```python
from build123d import *

# Parameters (mm, degrees)
SKETCH1_W                  = 44.45
SKETCH1_H                  = 44.45
BOSS_EXTRUDE1_DEPTH        = 9.525
CBORE_FOR_1_4_1_AT_2_COUNT = 2
CBORE_FOR_1_4_1_AT_2_PITCH = 45.963472584
CBORE_FOR_1_4_1_AT_3_COUNT = 2
CBORE_FOR_1_4_1_AT_3_PITCH = 32.501083151
SKETCH6_R                  = 6.35
CUT_EXTRUDE1_DEPTH         = 4.7752
SKETCH7_R                  = 2.38125
CUT_EXTRUDE2_DEPTH         = 33.842455374


with BuildPart() as part:
    # Sketch1 → Boss-Extrude1 (new body)
    with BuildSketch(Plane.XY):
        Rectangle(SKETCH1_W, SKETCH1_H)
    extrude(amount=BOSS_EXTRUDE1_DEPTH)

    # Sketch5 → CBORE for 1/4 _1 (revolve, cut)
    with BuildSketch(Plane(origin=(-15.875, 16.626083151, 0), x_dir=(0, 1, 0), z_dir=(1, 0, 0))):
        Polygon((0, 0), (0, 9.525), (3.175, 9.525), (3.175, 0.508), (3.81, 0.508), (3.81, 0.127), (3.937, 0), align=None)
    cbore_for_1_4_1 = revolve(axis=Axis((-15.875, 16.626083151, -6.35), (0, 0, 1)), mode=Mode.SUBTRACT)

    # CBORE for 1/4 _1 at 2: CBORE for 1/4 _1 ×2
    with Locations(*[Vector(0.7071067811865476, -0.7071067811865476, 0) * (i * CBORE_FOR_1_4_1_AT_2_PITCH) for i in range(1, CBORE_FOR_1_4_1_AT_2_COUNT)]):
        add(cbore_for_1_4_1, mode=Mode.SUBTRACT)

    # CBORE for 1/4 _1 at 3: CBORE for 1/4 _1 ×2
    with Locations(*[(0, -i * CBORE_FOR_1_4_1_AT_3_PITCH, 0) for i in range(1, CBORE_FOR_1_4_1_AT_3_COUNT)]):
        add(cbore_for_1_4_1, mode=Mode.SUBTRACT)

    # Sketch6 → Cut-Extrude1 (cut)
    with BuildSketch(Plane(origin=(0, 0, 0), x_dir=(-1, 0, 0), z_dir=(0, 0, -1))):
        with Locations((6.355653141, -6.355653141)):
            Circle(SKETCH6_R)
    extrude(amount=-CUT_EXTRUDE1_DEPTH, mode=Mode.SUBTRACT)

    # Sketch7 → Cut-Extrude2 (cut, through all)
    with BuildSketch(Plane(origin=(0, 0, 0), x_dir=(-1, 0, 0), z_dir=(0, 0, -1))):
        with Locations((6.355653141, -6.355653141)):
            Circle(SKETCH7_R)
    extrude(amount=-CUT_EXTRUDE2_DEPTH, mode=Mode.SUBTRACT)


solid = part.part
```
Here's how the part is built. I have some questions about the finished solid (model axes, mm). A direction names the side the tool comes from. Give positions to 0.01 mm unless a question says otherwise; leave off trailing zeros. Loops run counter-clockwise (first coordinate to the right, second up) from the corner with the lowest first, then second, coordinate; pieces in that order, holes last. Notation, with made-up numbers: M -22,32 L 35,32 A5 cw 35,40 Z; hole C -33,48.25 d10. An arc over 180 degrees is marked long. Return JSON: item names as keys, results as strings.
Item 1: On a 3-axis mill with a long thin cutter (end or side, diameter ignored), from which of +Z, -Z, +X, -X, +Y, -Y can I reach the whole of each face in a straight line? I mean faces 1 (the flat face through (14, -18, 0.508)), 2 (the flat face through (0, 0, 9.525)). Say none if no direction works.
A:
{"face 1": "-Z", "face 2": "+Z, +X, -X, +Y, -Y"}
Item 2: Please list where these lines run through material, in increasing order: line 1 (Y direction, x = -14, z = 2.75) (3 decimals); line 2 (Y direction, x = -17, z = 2) (3 decimals); line 3 (Y direction, x = 16.5, z = 1) (1 decimal).
A:
{"line 1": "y = -22.225 to -18.437, -13.313 to 14.064, 19.188 to 22.225", "line 2": "y = -22.225 to -18.844, -12.906 to 13.657, 19.595 to 22.225", "line 3": "y = -22.2 to -19, -12.7 to 22.2"}
Item 3: Imagine slicing it at B-B on z = 1.5. List the corners of the cut face in (x, y) for me (3 decimals), then the cut area to 3 significant figures.
A:
{"outline": "M -22.225,-22.225 L 22.225,-22.225 L 22.225,22.225 L -22.225,22.225 Z; hole C -15.875,-15.875 d6.35; hole C -15.875,16.626 d6.35; hole C -6.356,-6.356 d12.7; hole C 16.626,-15.875 d6.35", "area": "1,750 mm^2"}
Item 4: Imagine slicing it at C-C on y = -17.5. State how many separate pieces and enclosed holes the cut face has, then the cut area to 3 significant figures.
A:
{"separate pieces": "3", "enclosed holes": "0", "area": "318 mm^2"}
Item 5: Imagine slicing it at A-A on x = -4.5. List the corners of the cut face in (y, z) for me (3 decimals).
A:
{"outline": "M -22.225,0 L -12.428,0 L -12.428,4.775 L -7.848,4.775 L -7.848,9.525 L -22.225,9.525 Z; M -4.863,4.775 L -0.283,4.775 L -0.283,0 L 22.225,0 L 22.225,9.525 L -4.863,9.525 Z"}
Item 6: Thinking about a two-plate mould opening in X: for faces 3 (the flat face through (0, -22.225, 5)), 4 (the flat face through (22.225, 0, 5)), 5 (the cylindrical face through (-16.015, 13.454, 4.953)), which applies, released by +X, released by -X, zero draft, split by the parting line, or undercut?
A:
{"face 3": "zero draft", "face 4": "released by +X", "face 5": "undercut"}
Item 7: I'm going to push flat-ended pins straight in: pin 1 Ø10 at (x, y) = (-4, -5.5) entering from -Z; pin 2 Ø5 at (x, y) = (16.63, -15.88) entering from -Z; pin 3 Ø7.5 at (x, y) = (-6.36, -6.36) entering from -Z. Where does each tip first touch, or does it pass through?
A:
{"pin 1": "stops at z = 0", "pin 2": "passes through", "pin 3": "stops at z = 4.78"}
